Autodesk Inventor part; units mm, degrees
ref_plane "Work Plane1" through (-7.3154, 0, 0) normal (0, 0, -1) x (-1, 0, 0)
ref_plane "YZ Plane" through (0, 0, 0) normal (1, 0, 0) x (0, 1, 0)
ref_plane "XZ Plane" through (0, 0, 0) normal (0, 1, 0) x (-1, 0, 0)
sketch "Sketch1" plane through (0, 0, 0) normal (0, 1, 0) x (-1, 0, 0)
  circle A0 centre (0, 0) radius 4.125
  circle A1 centre (0, 0) radius 10.125
  line L0 (4.002, 1) -> (18.002, 1)
  line L1 (18.002, 1) -> (18.002, 7)
  line L2 (18.002, 7) -> (4.002, 7)
  line L3 (4.002, 7) -> (4.002, 1)
  line L4 (-15, 0) -> (15, 0) construction
  line L5 (-15, 0) -> (15, 0) construction
  line L6 (4.002, -1) -> (18.002, -1)
  line L7 (18.002, -1) -> (18.002, -7)
  line L8 (18.002, -7) -> (4.002, -7)
  line L9 (4.002, -7) -> (4.002, -1)
  point P0 (7.3154, 7)
  point P1 (7.3154, -7)
  point P2 (10.0755, -1)
  point P3 (4.0946, -5.2082)
  point P4 (4.002, -1)
  point P5 (4.0946, 5.2082)
  point P6 (10.0755, 1)
  dimension "eje" = 8.25
  dimension "diam_externo" = 20.25
  dimension "sep" = 1
  dimension "guia_central" = 30
  dimension "d4" = 0
  dimension "lengueta_espesor" = 6
  dimension "lengueta_alto" = 14
extrude "abrazadera" add sketch "Sketch1" along normal blind 15 contours L3 L2 A1 L0 | A0 L9 L8 A1 L2 L3 | L6 A1 L8 L9 | A1 L2 L1 L0 | L6 L7 L8 A1
sketch "Sketch5" plane through (-7.3154, 0, -7) normal (0, 0, -1) x (-1, 0, 0)
  circle A0 centre (3.6865, 7.6408) radius 2.075
  line L0 (-3.3135, 0) -> (-3.3135, 15)
  point P0 (-7.3154, 0)
  dimension "hueco_tornillo" = 4.15
  dimension "hueco_tornillo_distancia" = 7
extrude "tornillo" cut sketch "Sketch5" against normal blind 14
sketch "Sketch6" plane through (-7.3154, 0, -7) normal (0, 0, -1) x (-1, 0, 0)
  circle A0 centre (3.6865, 7.6408) radius 2.075
  circle A1 centre (3.6865, 7.6408) radius 5.5
  point P0 (-7.3154, 0)
  dimension "arandela" = 11
extrude "arandela" cut sketch "Sketch6" along normal blind 5 and the other way blind 1
ref_plane "Work Plane1" through (-7.3154, 0, 0) normal (0, 0, -1) x (-1, 0, 0)
mirror "Mirror1" about plane through (-7.3154, 0, 0) normal (0, 0, -1) of "arandela"
equation "\"diam_externo\" = eje + 2 * espesor"
equation "\"lengueta_espesor\" = espesor"
equation "\"hueco_tornillo_agujero\" = 2 * sep + 2 * lengueta_espesor"
equation "\"espesor\" = 6"
properties part number "Abrazadera"
Geometry check sheet. Reference: the model listing, model coordinates, mm. A direction names the side the tool comes from. Coordinates: 2 decimals unless noted, no trailing zeros. Order: outer loops, then holes, each group sorted by start corner. A loop starts at its lowest first (then second) coordinate and runs counter-clockwise, first axis right, second up. Notation, with made-up numbers: (70, 48) - (120, 48) arc R27 ccw to (120, 75) - close; hole circle Ø3 at (86, -26). An arc over 180 degrees is marked (long way). Answer in a Markdown table with one row per item. Add a question column.
1) Release check for a two-part mould opening along Y. For faces 1 (the flat face through (-4, 0, 2)), 2 (the flat face through (-4, 15, 2)), 3 (the flat face through (-13.4, 7.7, -6)) record: +Y half, -Y half, draft (parallel to the pull), parting line (faces both ways), or undercut.
2) Cross-section at B-B, the plane z = -3. Record the cut outline in (x, y) (3 decimals).
3) Set-up check for faces 4 (the flat face through (-17, 7, -7)), 5 (the flat face through (-9, 6, -1)), 6 (the cylindrical face through (-5.507, 7.399, 6.712)): record each of +Z, -Z, +X, -X, +Y, -Y from which the full face is reachable in a straight line by a thin tool's end or side.
4) Cross-section at A-A, the plane x = 0. Record the cut outline in (y, z) (3 decimals), then the cut area to 3 significant figures.
5) Cross-section at D-D, the plane x = -15. Record the cut outline in (y, z), then the cut area to 3 significant figures.
6) Cross-section at C-C, the plane z = -5.25. Record the cut outline in (x, y) (3 decimals), then the cut area to 3 significant figures.
7) Gauge pin test, flat ends, axial feed: P1, Ø1, axis at x = -7, y = 6.5, coming from the -Z side; P2, Ø5, axis at y = 13, z = -7.5, coming from the +X side; P3, Ø8.5, axis at x = -15, y = 8, coming from the -Z side; P4, Ø3.5, axis at x = -11, y = 7.64, coming from the -Z side. Record the tip position at first contact, or that the pin passes through.
8) Material ranges on line 1 along Z through (x, y) = (-15.75, 5.5); line 2 along Z through (x, y) = (-14.5, 2.5); line 3 along X through (y, z) = (9.5, 1.75), recorded low to high. Write a range as [from, to].
Check result:
| question | item | result |
|---|---|---|
| 1 | face 1 | -Y half |
| 1 | face 2 | +Y half |
| 1 | face 3 | undercut |
| 2 | outline | (-18.002, 0) - (-2.831, 0) - (-2.831, 15) - (-18.002, 15) - close; (2.831, 0) - (9.67, 0) - (9.67, 15) - (2.831, 15) - close; hole circle Ø4.15 at (-11.002, 7.641) |
| 3 | face 4 | -Z, -X, +Y, -Y |
| 3 | face 5 | -X, +Y, -Y |
| 3 | face 6 | +Z |
| 4 | outline | (0, -10.125) - (15, -10.125) - (15, -4.125) - (0, -4.125) - close; (0, 4.125) - (15, 4.125) - (15, 10.125) - (0, 10.125) - close |
| 4 | area | 180 mm² |
| 5 | outline | (0, -7) - (3.86, -7) - (3.86, -6) - (11.42, -6) - (11.42, -7) - (15, -7) - (15, -1) - (0, -1) - close; (0, 1) - (15, 1) - (15, 7) - (11.42, 7) - (11.42, 6) - (3.86, 6) - (3.86, 7) - (0, 7) - close |
| 5 | area | 165 mm² |
| 6 | outline | (-18.002, 0) - (8.658, 0) - (8.658, 15) - (-18.002, 15) - close; hole circle Ø4.15 at (-11.002, 7.641) |
| 6 | area | 386 mm² |
| 7 | P1 | stops at z = -6 |
| 7 | P2 | stops at x = 8.8 |
| 7 | P3 | stops at z = -7 |
| 7 | P4 | passes through |
| 8 | line 1 | z = [-6, -1], [1, 6] |
| 8 | line 2 | z = [-7, -1], [1, 7] |
| 8 | line 3 | x = [-18, -11.92], [-10.08, -3.74], [3.74, 9.97] |
